Here's the drawing with two shaded views (mm, measured from the low corner). I have some questions. Coordinates: 2 decimals unless noted, no trailing zeros. Loops run counter-clockwise (first coordinate to the right, second up) from the corner with the lowest first, then second, coordinate; pieces in that order, holes last. Notation, with made-up numbers: (6, 73) - (25, 73) arc R27 cw to (25, 108) - close; hole circle Ø9 at (13.25, 47.5). An arc over 180 degrees is marked (long way). One line per item, written item: value. Start each with the question number.
(1) If we section it at B-B on z = 103: Write out the boundary of the cut face in (x, y), then the cut area to 3 significant figures.
(2) If we section it at A-A on x = 4.25: Write out the boundary of the cut face in (y, z).
(3) If I drill on line 1 along Z through (x, y) = (0.75, 2.5); line 2 along X through (y, z) = (4, 47) (1 decimal); line 3 along Y through (x, z) = (2.5, 134), over which ranges is the centre line in solid material (lowest first)? Write a range as from..to.
(4) I'm going to push flat-ended pins straight in: P1, Ø1.5, axis at x = 3.5, z = 103, coming from the -Y side; P2, Ø1, axis at x = 1.5, z = 83.5, coming from the +Y side (1 decimal); P3, Ø3, axis at y = 3.5, z = 133, coming from the +X side. Where does each tip first touch, or does it pass through?
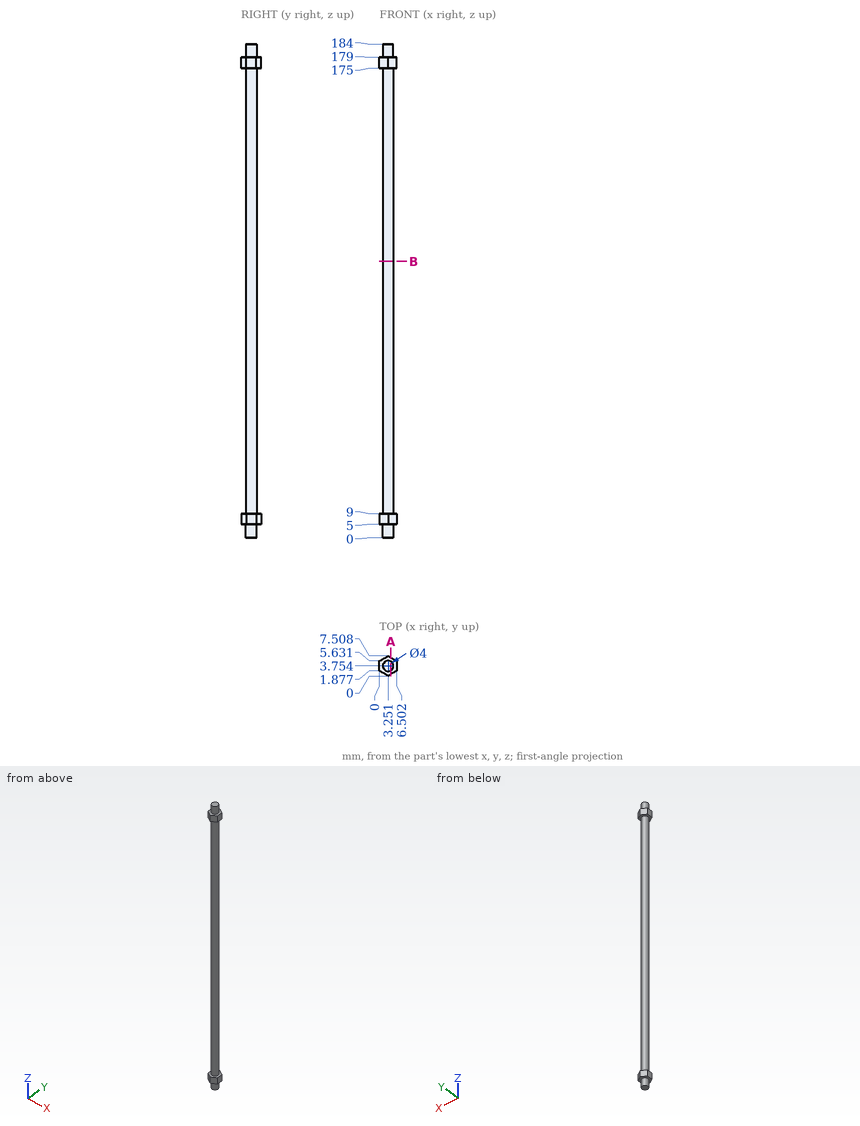
Values:
1. outline: circle Ø4 at (3.25, 3.75)
1. area: 12.6 mm2
2. outline: (0.58, 5) - (2.02, 5) - (2.02, 0) - (5.49, 0) - (5.49, 5) - (6.93, 5) - (6.93, 9) - (5.49, 9) - (5.49, 175) - (6.93, 175) - (6.93, 179) - (5.49, 179) - (5.49, 184) - (2.02, 184) - (2.02, 179) - (0.58, 179) - (0.58, 175) - (2.02, 175) - (2.02, 9) - (0.58, 9) - close
3. line 1: z = 5..9, 175..179
3. line 2: x = 1.3..5.2
3. line 3: y = 1.9..5.61
4. P1: stops at y = 1.75
4. P2: stops at y = 5.3
4. P3: stops at x = 5.25
